from build123d import *

# Parameters (mm, degrees)
F1_ANGLE = 180


with BuildPart() as f1:
    # F0 (on Top) → F1 (revolve)
    with BuildSketch(Plane.XY):
        Polygon((-9.93075, 8.25), (-9.93075, 3.75), (-8.13075, 3.75), (-8.13075, 5), (2.56925, 5), (2.56925, 6.65), (6.66925, 6.65), (6.66925, 5), (7.86925, 5), (7.86925, 10), (-8.13075, 10), (-53.43075, 10), (-53.43075, 7.2), (-50.93075, 7.2), (-50.93075, 8), (-24.43075, 8), (-24.43075, 8.25), align=None)
    revolve(axis=Axis((-13.705372, 0, 0), (-1, 0, 0)), revolution_arc=F1_ANGLE)


solid = f1.part
The listing builds one solid part. Answer for the finished solid, in the listing's coordinates (mm). A direction names the side the tool comes from. Coordinates: 2 decimals unless noted, no trailing zeros. Loops run counter-clockwise (first coordinate to the right, second up) from the corner with the lowest first, then second, coordinate; pieces in that order, holes last. Notation, with made-up numbers: (44.5, 0) -> (62.5, 0) arc R25 ccw to (62.5, 19) -> close; hole circle Ø11 at (53, -5). An arc over 180 degrees is marked (long way). Answer in a Markdown table with one row per item. Add a question column.
1. The part is cut by section C-C, the plane x = -25.5. Write down the section's boundary in (y, z).
2. The part is cut by section D-D, the plane y = 2.75. Write down the section's boundary in (x, z), then the cut area to 3 significant figures.
3. For faces 1 (the cylindrical face through (-37, 0, -8)), 2 (the flat face through (7.869, 0, -6)), 3 (the cylindrical face through (-23, 0, -10)), 4 (the cylindrical face through (-52.16, 0.16, -7.2)), 5 (the cylindrical face through (-3, 0, -5)), determine the directions among +Z, -Z, +X, -X, +Y, -Y from which every point of the face is accessible in a straight line to the end or side of a thin tool.
4. The part is cut by section A-A, the plane y = 0. Write down the section's boundary in (x, z).
5. Determine the mould class of faces 6 (the flat face through (-53.431, -2.4, -7.3)), 7 (the flat face through (-50.931, 1.2, -7.3)), 8 (the flat face through (-16, 9, 0)), 9 (the flat face through (6.669, 0, -6)) for opening direction X: +X half, -X half, draft (parallel to the pull), parting line (faces both ways), or undercut.
6. Flat-ended cylindrical pins translate along their axes: P1, Ø2.5, axis at y = -1, z = -2, coming from the +X side; P2, Ø2, axis at x = 0, z = -1.5, coming from the +Y side; P3, Ø2, axis at x = -21, z = -8, coming from the -Y side; P4, Ø2.5, axis at y = 2, z = -2, coming from the +X side. Find the tip coordinate at first contact, or state that the pin passes through.
7. Consider line 1 (X direction, y = 3, z = -5.75); line 2 (Y direction, x = -19, z = -1.75); line 3 (X direction, y = -2.75, z = -6.75). Determine where each line is inside the solid, lowest interval first. Write a range as [from, to].
8. The part is cut by section B-B, the plane z = -6. Write down the section's boundary in (x, y), then the cut area to 3 significant figures.
Answer below:
| question | item | result |
|---|---|---|
| 1 | outline | (-10, 0) arc R10 ccw to (10, 0) -> (8, 0) arc R8 cw to (-8, 0) -> close |
| 2 | outline | (-53.43, -9.61) -> (7.87, -9.61) -> (7.87, -4.18) -> (6.67, -4.18) -> (6.67, -6.05) -> (2.57, -6.05) -> (2.57, -4.18) -> (-8.13, -4.18) -> (-8.13, -2.55) -> (-9.93, -2.55) -> (-9.93, -7.78) -> (-24.43, -7.78) -> (-24.43, -7.51) -> (-50.93, -7.51) -> (-50.93, -6.65) -> (-53.43, -6.65) -> close |
| 2 | area | 182 mm2 |
| 3 | face 1 | +Z |
| 3 | face 2 | +Z, -Z, +X, +Y, -Y |
| 3 | face 3 | -Z, +X, -X |
| 3 | face 4 | +Z, -X |
| 3 | face 5 | +Z, +X |
| 4 | outline | (-53.43, -10) -> (7.87, -10) -> (7.87, -5) -> (6.67, -5) -> (6.67, -6.65) -> (2.57, -6.65) -> (2.57, -5) -> (-8.13, -5) -> (-8.13, -3.75) -> (-9.93, -3.75) -> (-9.93, -8.25) -> (-24.43, -8.25) -> (-24.43, -8) -> (-50.93, -8) -> (-50.93, -7.2) -> (-53.43, -7.2) -> close |
| 5 | face 6 | -X half |
| 5 | face 7 | undercut |
| 5 | face 8 | draft |
| 5 | face 9 | undercut |
| 6 | P1 | through |
| 6 | P2 | y = 9.99 |
| 6 | P3 | y = -7.14 |
| 6 | P4 | x = -8.13 |
| 7 | line 1 | [-9.93, 2.57], [6.67, 7.87] |
| 7 | line 2 | [-9.85, -8.06], [8.06, 9.85] |
| 7 | line 3 | [-53.43, -50.93], [-9.93, 7.87] |
| 8 | outline | (-53.43, -8) -> (7.87, -8) -> (7.87, 8) -> (-53.43, 8) -> (-53.43, 3.98) -> (-50.93, 3.98) -> (-50.93, 5.29) -> (-24.43, 5.29) -> (-24.43, 5.66) -> (-9.93, 5.66) -> (-9.93, -5.66) -> (-24.43, -5.66) -> (-24.43, -5.29) -> (-50.93, -5.29) -> (-50.93, -3.98) -> (-53.43, -3.98) -> close; hole (2.57, -2.87) -> (6.67, -2.87) -> (6.67, 2.87) -> (2.57, 2.87) -> close |
| 8 | area | 493 mm2 |
